from build123d import *

# Parameters (mm, degrees)
F2_R     = 1.25
F3_DEPTH = 2
F4_SIZE  = 0.3


with BuildPart() as f1:
    # F0 (on Front) → F1 (revolve)
    with BuildSketch(Plane.XZ):
        Polygon((0, -15), (0, 0), (-4, 0), (-3, -15), align=None)
    revolve(axis=Axis((0, 0, -6.756781), (0, 0, -1)))

    # F2 (on face) → F3 (join)
    with BuildSketch(Plane.XY):
        Circle(F2_R)
    extrude(amount=F3_DEPTH)

    # F4
    f4_edges = [f1.edges().sort_by_distance(p)[0] for p in [
        (-1.25, 0, 2),
    ]]
    chamfer(f4_edges, length=F4_SIZE)


solid = f1.part
Part model, mm, in its own coordinate system. A direction names the side the tool comes from. Give positions to 0.01 mm unless a question says otherwise; leave off trailing zeros. Order: outer loops, then holes, each group sorted by start corner. A loop starts at its lowest first (then second) coordinate and runs counter-clockwise, first axis right, second up. Notation, with made-up numbers: (15.25, 56.25) - (33.25, 56.25) arc R20 ccw to (33.25, 87.25) - close; hole circle Ø6 at (-21.75, 33). An arc over 180 degrees is marked (long way). Use a Markdown table: item, result.
1) Saw through at C-C on z = -8.25. List the corners of the cut face in (x, y), plus the area to 3 significant figures.
Checked values:
| item | result |
|---|---|
| outline | circle Ø6.9 at (0, 0) |
| area | 37.4 mm² |
2) Saw through at A-A on x = 0. List the corners of the cut face in (y, z), plus the area to 3 significant figures.
Checked values:
| item | result |
|---|---|
| outline | (-4, 0) - (-3, -15) - (3, -15) - (4, 0) - (1.25, 0) - (1.25, 1.7) - (0.95, 2) - (-0.95, 2) - (-1.25, 1.7) - (-1.25, 0) - close |
| area | 110 mm² |
3) Flat gauge pins, fed straight in: P1, Ø1.5, axis at x = 3, z = -11.5, coming from the +Y side; P2, Ø2, axis at y = -2, z = -0.5, coming from the +X side. Where does each tip first touch, or does it go through?
Checked values:
| item | result |
|---|---|
| P1 | y = 2.33 |
| P2 | x = 3.85 |
4) Probe L1, parallel to Z at x = 1.25, y = 1.25; L2, parallel to X at y = -2, z = -4.5; L3, parallel to Y at x = -1, z = -8. List the from-to ranges inside material, lowest first. Write a range as from..to.
Checked values:
| item | result |
|---|---|
| L1 | -15..0 |
| L2 | -3.11..3.11 |
| L3 | -3.32..3.32 |
5) 3-axis set-ups, long thin cutter, end or side, ignore diameter. For faces 1 (the flat face through (0, 0, 2)), 2 (the cylindrical face through (-0.27, -1.22, 0.84)): which of +Z, -Z, +X, -X, +Y, -Y reach the whole face in a straight line?
Checked values:
| item | result |
|---|---|
| face 1 | +Z, +X, -X, +Y, -Y |
| face 2 | +Z |
6) Saw through at D-D on z = -3. List the corners of the cut face in (x, y), plus the area to 3 significant figures.
Checked values:
| item | result |
|---|---|
| outline | circle Ø7.6 at (0, 0) |
| area | 45.4 mm² |
